Can you work these out from the drawing? Everything is in mm from the part's minimum corner. Coordinates: 2 decimals unless noted, no trailing zeros. Loops run counter-clockwise (first coordinate to the right, second up) from the corner with the lowest first, then second, coordinate; pieces in that order, holes last. Notation, with made-up numbers: (53, -19.75) -> (71, -19.75) arc R17 ccw to (71, 0.25) -> close; hole circle Ø1 at (29, -36). An arc over 180 degrees is marked (long way). Use one line per item in the form item = value. Start each with the question number.
(1) I'm going to push a flat-ended pin straight in: pin 1 (1.5 mm diameter, centred on x = 0.5, y = 34, fed in from -Z). Where does the tip first touch, or does it pass through?
(2) I need wall thicknesses on line 1 (Y direction, x = 0.5, z = 3.5); line 2 (Y direction, x = 2, z = 9.75); line 3 (Z direction, x = 0.1, y = 35). Which ranges of each line are inside material? Lowest first, please. Write a range as [from, to].
(3) Imagine slicing it at C-C (y = 33.5). List the corners of the cut face in (x, z) for me.
(4) Imagine slicing it at B-B (z = 7). List the corners of the cut face in (x, y) for me, plus the area to 3 significant figures.
(5) Imagine slicing it at A-A (x = 0.95). List the corners of the cut face in (y, z) for me, plus the area to 3 significant figures.
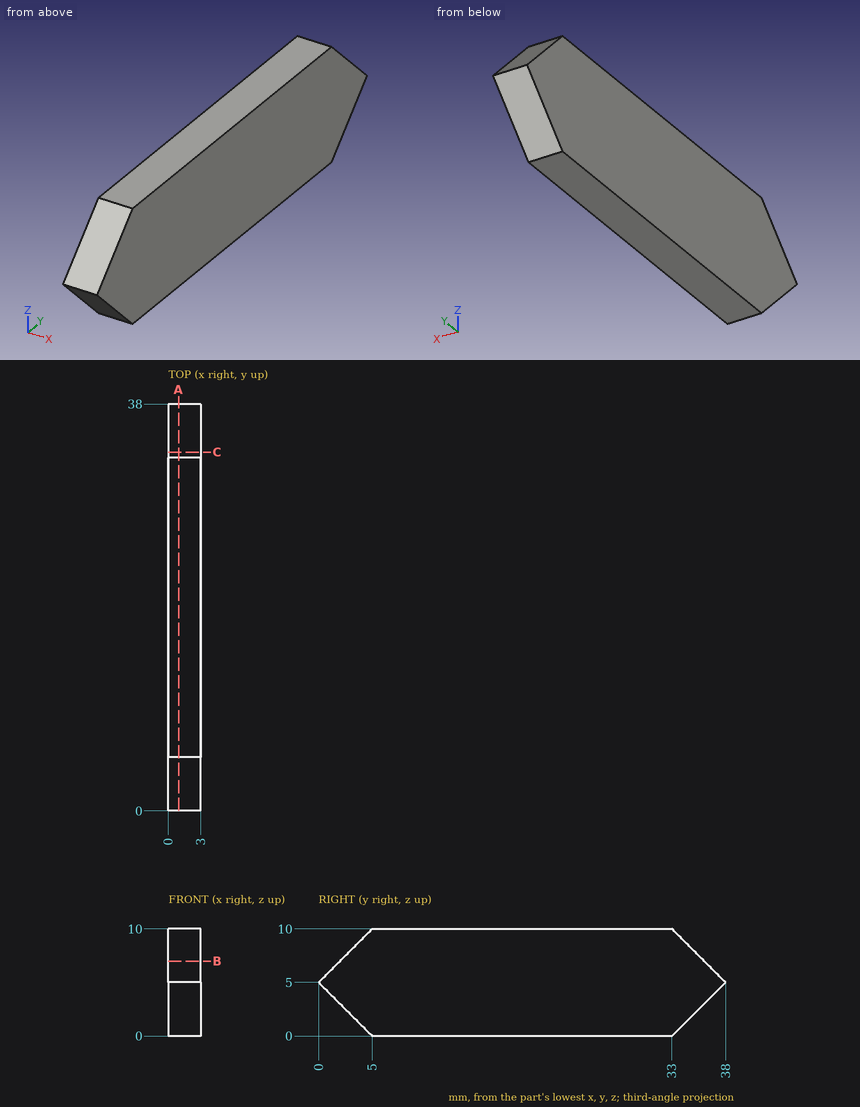
Worked out:
q1.pin_1 = 0.25
q2.line_1 = [1.5, 36.5]
q2.line_2 = [4.75, 33.25]
q2.line_3 = [2, 8]
q3.outline = (0, 0.5) -> (3, 0.5) -> (3, 9.5) -> (0, 9.5) -> close
q4.outline = (0, 2) -> (3, 2) -> (3, 36) -> (0, 36) -> close
q4.area = 102 mm2
q5.outline = (0, 5) -> (5, 0) -> (33, 0) -> (38, 5) -> (33, 10) -> (5, 10) -> close
q5.area = 330 mm2
